Design review of the part built by this model. Coordinates are the model's own, in mm. Face numbers are marked on the shaded views. A direction names the side the tool comes from. Coordinates: 2 decimals unless noted, no trailing zeros. Loops run counter-clockwise (first coordinate to the right, second up) from the corner with the lowest first, then second, coordinate; pieces in that order, holes last. Notation, with made-up numbers: (-35, 26) -> (-3, 26) arc R19 cw to (-3, 43) -> close; hole circle Ø10 at (37, 75). An arc over 180 degrees is marked (long way). Answer in a Markdown table with one row per item.
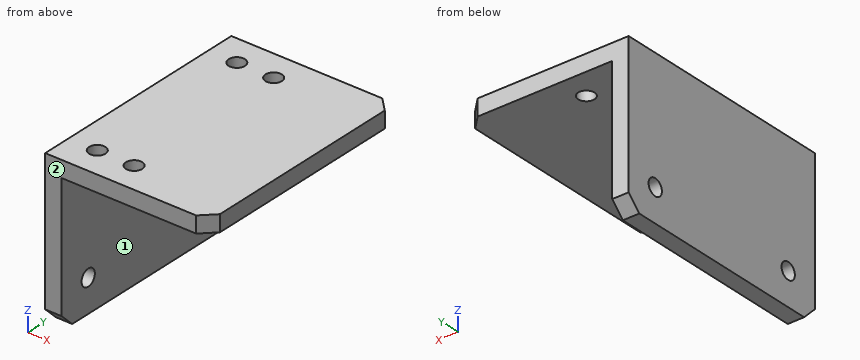
```python
from build123d import *

# Parameters (mm, degrees)
F1_DEPTH = 88.9
F3_D     = 6.35
F4_SIZE  = 5.08
F6_D     = 6.35


with BuildPart() as f1:
    # F0 (on Front) → F1 (new body)
    with BuildSketch(Plane.XZ):
        Polygon((27.723321, 33.983968), (-29.426679, 33.983968), (-35.776679, 33.983968), (-35.776679, -25.72097), (-29.426679, -25.72097), (-29.426679, 27.633968), (27.723321, 27.633968), align=None)
    extrude(amount=F1_DEPTH)

    # F3 (through all)
    with Locations(Plane.YZ.offset(-29.426679)):
        with Locations((-76.2, -13.02097), (-12.7, -13.02097)):
            Hole(F3_D / 2)

    # F4
    f4_edges = [f1.edges().sort_by_distance(p)[0] for p in [
        (-32.601679, -88.9, -25.72097),
        (27.723321, -88.9, 30.808968),
        (27.723321, 0, 30.808968),
        (-32.601679, 0, -25.72097),
    ]]
    chamfer(f4_edges, length=F4_SIZE)

    # F6 (through all)
    with Locations(Plane.XY.offset(33.983968)):
        with Locations((-10.376679, -11.1252), (-24.651479, -11.1252), (-24.651479, -77.7748), (-10.376679, -77.7748)):
            Hole(F6_D / 2)


solid = f1.part
```
(1) For pin 1 (5 mm diameter, centred on x = -7, z = 23, fed in from +Y); pin 2 (12 mm diameter, centred on x = -12.5, y = -73.5, fed in from -Z); pin 3 (8.5 mm diameter, centred on y = -12.7, z = -13.02, fed in from +X), all flat-tipped, find the tip position at first contact; note any pin that passes through.
Evaluation:
| item | result |
|---|---|
| pin 1 | passes through |
| pin 2 | stops at z = 27.63 |
| pin 3 | stops at x = -29.43 |
(2) To check wall thickness, follow probe 1 along Z at (x, y) = (-32, -12.7); probe 2 along Z at (x, y) = (-7, -43.5); probe 3 along X at (y, z) = (-35, -10.5). State the ranges of each line that lie inside material, in increasing order.
Evaluation:
| item | result |
|---|---|
| probe 1 | z = -25.72 to -16.2, -9.85 to 33.98 |
| probe 2 | z = 27.63 to 33.98 |
| probe 3 | x = -35.78 to -29.43 |
(3) Tool access review of the marked faces 1 and 2: name each direction out of +Z, -Z, +X, -X, +Y, -Y from which nothing blocks a thin tool from reaching the whole face with its end or side.
Evaluation:
| item | result |
|---|---|
| face 1 | -Z, +X, +Y, -Y |
| face 2 | +Z, -Z, +X, -X, -Y |
(4) Take a section at A-A on y = -76.2. Give the boundary of the cut face in (x, z).
Evaluation:
| item | result |
|---|---|
| outline | (-35.78, -25.72) -> (-29.43, -25.72) -> (-29.43, -16.2) -> (-35.78, -16.2) -> close; (-35.78, -9.85) -> (-29.43, -9.85) -> (-29.43, 27.63) -> (-27.41, 27.63) -> (-27.41, 33.98) -> (-35.78, 33.98) -> close; (-21.89, 27.63) -> (-13.13, 27.63) -> (-13.13, 33.98) -> (-21.89, 33.98) -> close; (-7.62, 27.63) -> (27.72, 27.63) -> (27.72, 33.98) -> (-7.62, 33.98) -> close |
(5) Take a section at D-D on x = 3.5. Give the boundary of the cut face in (y, z), and give its area (3 significant figures).
Evaluation:
| item | result |
|---|---|
| outline | (-88.9, 27.63) -> (0, 27.63) -> (0, 33.98) -> (-88.9, 33.98) -> close |
| area | 565 mm² |
(6) Take a section at C-C on y = -32. Give the boundary of the cut face in (x, z).
Evaluation:
| item | result |
|---|---|
| outline | (-35.78, -25.72) -> (-29.43, -25.72) -> (-29.43, 27.63) -> (27.72, 27.63) -> (27.72, 33.98) -> (-35.78, 33.98) -> close |
(7) Take a section at B-B on z = 6. Give the boundary of the cut face in (x, y).
Evaluation:
| item | result |
|---|---|
| outline | (-35.78, -88.9) -> (-29.43, -88.9) -> (-29.43, 0) -> (-35.78, 0) -> close |
